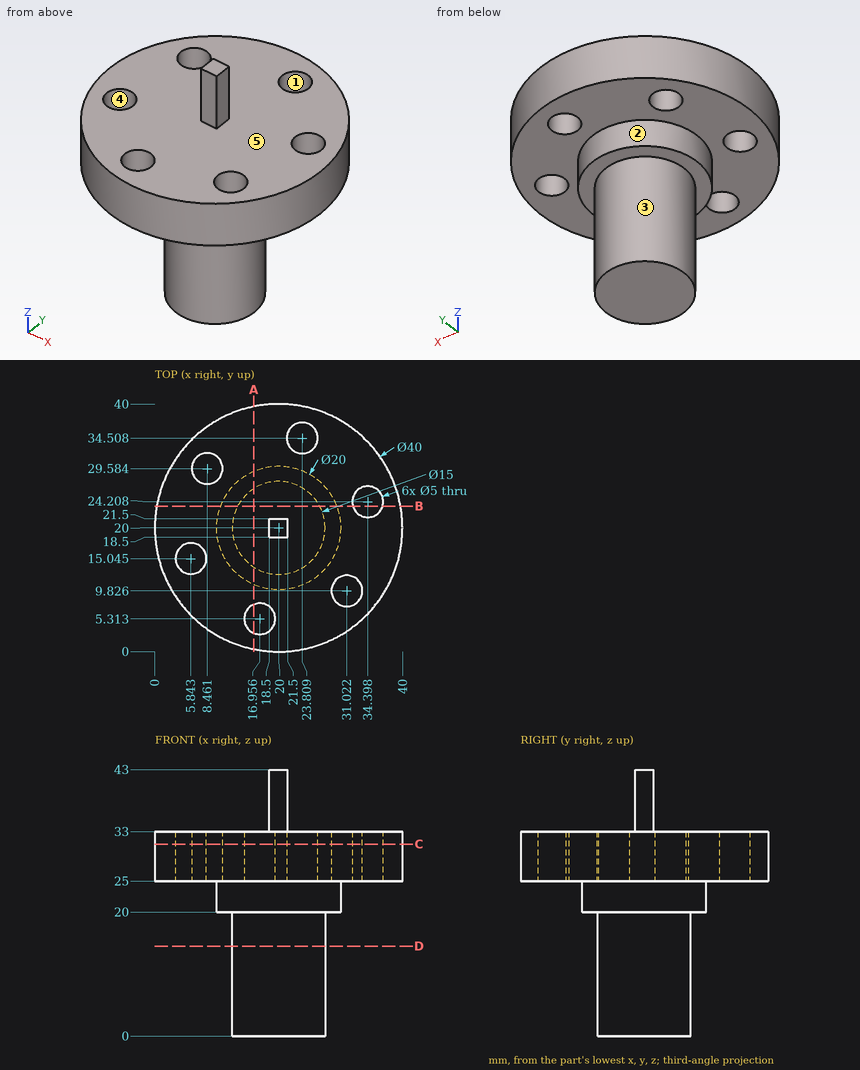
Can you work these out from the drawing? Everything is in mm from the part's minimum corner. A direction names the side the tool comes from. Coordinates: 2 decimals unless noted, no trailing zeros. Write each loop counter-clockwise with the first axis right and the second up, starting at its lowest first coordinate (ties: lowest second). Pieces come first, ordered by that corner, then holes. Notation, with made-up numbers: (-26.75, 33.25) -> (26.25, 33.25) arc R20 cw to (26.25, 59.25) -> close; hole circle Ø4 at (15, -32). An arc over 180 degrees is marked (long way). Return JSON: item names as keys, results as strings.
(1) Which directions (+Z, -Z, +X, -X, +Y, -Y) give clear straight access to the entire face, cutting with the end or side of a thin tool? Please do the marked faces 1 and 2.
Numbers:
{"face 1": "+Z, -Z", "face 2": "-Z"}
(2) I need wall thicknesses on L1, parallel to Z at x = 18, y = 33; L2, parallel to Z at x = 23, y = 20; L3, parallel to X at y = 25, z = 27 (1 decimal). Which ranges of each line are inside material? Lowest first, please.
Numbers:
{"L1": "z = 25 to 33", "L2": "z = 0 to 33", "L3": "x = 0.6 to 32, 36.8 to 39.4"}
(3) Imagine slicing it at B-B, the plane y = 23.5. Please give me the cut outline in (x, z) (1 decimal), then the cut area to 3 significant figures.
Numbers:
{"outline": "(0.3, 25) -> (10.6, 25) -> (10.6, 20) -> (13.4, 20) -> (13.4, 0) -> (26.6, 0) -> (26.6, 20) -> (29.4, 20) -> (29.4, 25) -> (32, 25) -> (32, 33) -> (0.3, 33) -> close; (36.8, 25) -> (39.7, 25) -> (39.7, 33) -> (36.8, 33) -> close", "area": "636 mm2"}
(4) We'd pull the mould along Y, two halves only. Please class the marked faces 3, 4 and 5: +Y half, -Y half, draft (parallel to the pull), parting line (faces both ways), or undercut.
Numbers:
{"face 3": "parting line", "face 4": "undercut", "face 5": "draft"}
(5) Imagine slicing it at A-A, the plane x = 16. Please give me the cut outline in (y, z) (1 decimal), then the cut area to 3 significant figures.
Numbers:
{"outline": "(0.4, 25) -> (3, 25) -> (3, 33) -> (0.4, 33) -> close; (7.6, 25) -> (10.8, 25) -> (10.8, 20) -> (13.7, 20) -> (13.7, 0) -> (26.3, 0) -> (26.3, 20) -> (29.2, 20) -> (29.2, 25) -> (39.6, 25) -> (39.6, 33) -> (7.6, 33) -> close", "area": "622 mm2"}
(6) I'm going to push flat-ended pins straight in: pin 1 (4.5 mm diameter, centred on x = 8.46, y = 29.58, fed in from -Z); pin 2 (6 mm diameter, centred on x = 23.5, z = 32.5, fed in from -Y); pin 3 (2.5 mm diameter, centred on y = 20.5, z = 39, fed in from +X); pin 4 (2.5 mm diameter, centred on y = 20, z = 36.5, fed in from -X). Where does each tip first touch, or does it pass through?
Numbers:
{"pin 1": "passes through", "pin 2": "stops at y = 0.01", "pin 3": "stops at x = 21.5", "pin 4": "stops at x = 18.5"}
(7) Imagine slicing it at D-D, the plane z = 14.5. Please give me the cut outline in (x, y).
Numbers:
{"outline": "circle Ø15 at (20, 20)"}
(8) Imagine slicing it at C-C, the plane z = 31. Please give me the cut outline in (x, y) (1 decimal), then the cut area to 3 significant figures.
Numbers:
{"outline": "circle Ø40 at (20, 20); hole circle Ø5 at (5.8, 15); hole circle Ø5 at (8.5, 29.6); hole circle Ø5 at (17, 5.3); hole circle Ø5 at (23.8, 34.5); hole circle Ø5 at (31, 9.8); hole circle Ø5 at (34.4, 24.2)", "area": "1,140 mm2"}
